from build123d import *

# Parameters (mm, degrees)
PAD_DEPTH = 10
FILLET_R  = 2


with BuildPart() as part:
    # Sketch → Pad (new body)
    with BuildSketch(Plane.XZ):
        with BuildLine():
            Line((-29.102787, 29.073721), (39.458904, 11.629483))
            ThreePointArc((39.458904, -11.629483), (48.5, 0), (39.458904, 11.629483))
            Line((-29.102787, -29.073721), (39.458904, -11.629483))
            ThreePointArc((-29.102787, 29.073721), (-66.5, 0), (-29.102787, -29.073721))
        make_face()
    extrude(amount=PAD_DEPTH)

    # Fillet
    fillet_edges = [part.edges().sort_by_distance(p)[0] for p in [
        (-66.5, -10, 0),
        (5.178059, -10, 20.351602),
        (48.5, -10, 0),
        (5.178059, -10, -20.351602),
        (-66.5, 0, 0),
        (5.178059, 0, 20.351602),
        (48.5, 0, 0),
        (5.178059, 0, -20.351602),
    ]]
    fillet(fillet_edges, radius=FILLET_R)


solid = part.part
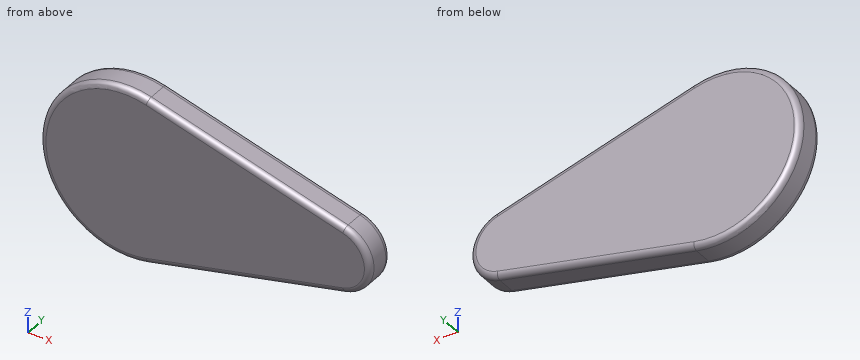
The model under review builds one solid part; all positions refer to its coordinate system, in mm. Give positions to 0.01 mm unless a question says otherwise; leave off trailing zeros. Write each loop counter-clockwise with the first axis right and the second up, starting at its lowest first coordinate (ties: lowest second). Pieces come first, ordered by that corner, then holes.
1. For P1, Ø5, axis at x = 27.5, y = -4, coming from the -Z side; P2, Ø1.5, axis at x = 1, y = -2.5, coming from the +Z side; P3, Ø2, axis at x = -55, y = -4.5, coming from the -Z side, all flat-tipped, find the tip position at first contact; note any pin that passes through.
2. Add section A-A, the plane y = -6. Write out the cut boundary in (x, z), plus the area to 3 significant figures.
3. Wall thickness on L1, parallel to Z at x = -37.5, y = -4; L2, parallel to X at y = -2.5, z = -1.5; L3, parallel to Z at x = -17, y = -6.5: over which ranges is each line inside the solid? List them lowest first.
Worked answers:
1. P1: stops at z = -15.31
1. P2: stops at z = 21.61
1. P3: stops at z = -24.37
2. outline: (-29.1, -29.07) - (39.46, -11.63) arc R12 ccw to (39.46, 11.63) - (-29.1, 29.07) arc R30 ccw (long way) to start
2. area: 4,800 mm2
3. L1: z = -29.98 to 29.98
3. L2: x = -66.46 to 48.41
3. L3: z = -25.99 to 25.99
